Read the model definition and answer for the solid it produces. Units are mm, in the model's axes. Face numbers are marked on the shaded views. Round coordinates to 2 decimals unless told otherwise and drop trailing zeros. Write each loop counter-clockwise with the first axis right and the second up, starting at its lowest first coordinate (ties: lowest second). Pieces come first, ordered by that corner, then holes. Notation, with made-up numbers: (36.5, 17.5) -> (49.5, 17.5) arc R33 ccw to (49.5, 56.5) -> close; hole circle Ø1 at (-1, 77.25). An arc over 180 degrees is marked (long way). Return JSON: item names as keys, results as strings. Group by question number.
(1) Given pin 1 (1.1 mm diameter, centred on y = 10, z = -21, fed in from +X); pin 2 (8 mm diameter, centred on y = 10.5, z = -39, fed in from +X); pin 3 (8 mm diameter, centred on x = -22.5, y = 11.5, fed in from -Z), each flat-ended and moving along its own axis, determine where each tip first touches the part or whether it passes through.
(2) Straight lines are drawn through the part: line 1 (Z direction, x = -39.5, y = 1); line 2 (X direction, y = 2.1, z = 0); line 3 (X direction, y = 10.5, z = -7.5). For each, find the intervals that lie inside material, in ascending order.
(3) A cutting plane is placed at A-A on z = 0. Give the vertices of the cut face in (x, y), then the cut area to 3 significant figures.
(4) A cutting plane is placed at D-D on x = -20. Give the vertices of the cut face in (y, z).
(5) A cutting plane is placed at B-B on x = -40. Give the vertices of the cut face in (y, z), then the cut area to 3 significant figures.
(6) The mould has two halves that part along Y. Classify the marked faces 1 and 2: released by +Y, released by -Y, zero draft, split by the parting line, or undercut.
(7) A cutting plane is placed at C-C on z = 46.4. Give the vertices of the cut face in (x, y), then the cut area to 3 significant figures.
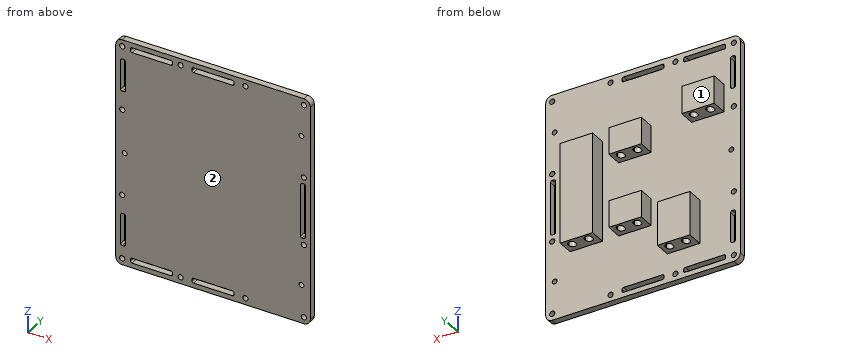
```python
from build123d import *

# Parameters (mm, degrees)
SKETCH1_W               = 120
SKETCH1_H               = 140
BOSS_EXTRUDE1_DEPTH     = 4
SKETCH2_R               = 1.6
CUT_EXTRUDE1_DEPTH      = 4
FILLET1_R               = 4
SKETCH5_W               = 20
SKETCH5_H               = 62
SKETCH5_H_2             = 27
BOSS_EXTRUDE2_DEPTH     = 10
SKETCH6_W               = 20
SKETCH6_H               = 10
SKETCH6_H_2             = 29
CUT_EXTRUDE3_DEPTH      = 10
CUT_EXTRUDE4_DEPTH      = 40
CUT_EXTRUDE4_DEPTH_BACK = 102
CUT_EXTRUDE5_DEPTH      = 20
CUT_EXTRUDE6_DEPTH      = 30
CUT_EXTRUDE7_DEPTH      = 5
SKETCH11_R              = 1.5
CUT_EXTRUDE8_DEPTH      = 5


with BuildPart() as part:
    # Sketch1 → Boss-Extrude1 (new body)
    with BuildSketch(Plane(origin=(0, 0, 0), x_dir=(1, 0, 0), z_dir=(0, 1, 0))):
        Rectangle(SKETCH1_W, SKETCH1_H)
    extrude(amount=BOSS_EXTRUDE1_DEPTH)

    # Sketch2 → Cut-Extrude1 (cut)
    with BuildSketch(Plane(origin=(0, 4, 0), x_dir=(1, 0, 0), z_dir=(0, 1, 0))):
        with Locations((-56, 66)):
            Circle(SKETCH2_R)
        with Locations((56, 66)):
            Circle(SKETCH2_R)
        with Locations((-56, -66)):
            Circle(SKETCH2_R)
        with Locations((56, -66)):
            Circle(SKETCH2_R)
        with Locations((-20, -66)):
            Circle(SKETCH2_R)
        with Locations((20, -66)):
            Circle(SKETCH2_R)
        with Locations((-20, 66)):
            Circle(SKETCH2_R)
        with Locations((20, 66)):
            Circle(SKETCH2_R)
        with Locations((-56, -26.5)):
            Circle(SKETCH2_R)
        with Locations((-56, 26.5)):
            Circle(SKETCH2_R)
        with Locations((56, -21)):
            Circle(SKETCH2_R)
        with Locations((56, 21)):
            Circle(SKETCH2_R)
    extrude(amount=-CUT_EXTRUDE1_DEPTH, mode=Mode.SUBTRACT)

    # Fillet1
    fillet1_edges = [part.edges().sort_by_distance(p)[0] for p in [
        (60, 2, 70),
        (-60, 2, 70),
        (-60, 2, -70),
        (60, 2, -70),
    ]]
    fillet(fillet1_edges, radius=FILLET1_R)

    # Sketch5 → Boss-Extrude2 (add)
    with BuildSketch(Plane(origin=(0, 4, 0), x_dir=(1, 0, 0), z_dir=(0, 1, 0))):
        with Locations((35, 0)):
            Rectangle(SKETCH5_W, SKETCH5_H)
        with Locations((-25, 38.5)):
            Rectangle(SKETCH5_W, SKETCH5_H_2)
        with Locations((5, 0)):
            Rectangle(SKETCH5_W, SKETCH5_H)
        with Locations((-40, -38.5)):
            Rectangle(SKETCH5_W, SKETCH5_H_2)
    extrude(amount=BOSS_EXTRUDE2_DEPTH)

    # Sketch6 → Cut-Extrude3 (cut)
    with BuildSketch(Plane(origin=(0, 14, 0), x_dir=(1, 0, 0), z_dir=(0, 1, 0))):
        with Locations((-40, -47)):
            Rectangle(SKETCH6_W, SKETCH6_H)
        with Locations((5, 0)):
            Rectangle(SKETCH6_W, SKETCH6_H_2)
    extrude(amount=-CUT_EXTRUDE3_DEPTH, mode=Mode.SUBTRACT)

    # Sketch7 → Cut-Extrude4 (cut, two sides)
    with BuildSketch(Plane.XY.offset(31)) as cut_extrude4_sk:
        with BuildLine():
            Line((-2.3, 9.4), (-2.3, 10.4))
            ThreePointArc((-2.3, 10.4), (-0.1, 12.6), (2.1, 10.4))
            Line((2.1, 10.4), (2.1, 9.4))
            ThreePointArc((2.1, 9.4), (-0.1, 7.2), (-2.3, 9.4))
        make_face()
        with BuildLine():
            Line((7.9, 9.4), (7.9, 10.4))
            ThreePointArc((7.9, 10.4), (10.1, 12.6), (12.3, 10.4))
            Line((12.3, 10.4), (12.3, 9.4))
            ThreePointArc((12.3, 9.4), (10.1, 7.2), (7.9, 9.4))
        make_face()
        with BuildLine():
            Line((27.7, 9.4), (27.7, 10.4))
            ThreePointArc((27.7, 10.4), (29.9, 12.6), (32.1, 10.4))
            Line((32.1, 10.4), (32.1, 9.4))
            ThreePointArc((32.1, 9.4), (29.9, 7.2), (27.7, 9.4))
        make_face()
        with BuildLine():
            Line((37.9, 9.4), (37.9, 10.4))
            ThreePointArc((37.9, 10.4), (40.1, 12.6), (42.3, 10.4))
            Line((42.3, 10.4), (42.3, 9.4))
            ThreePointArc((42.3, 9.4), (40.1, 7.2), (37.9, 9.4))
        make_face()
    extrude(amount=CUT_EXTRUDE4_DEPTH, mode=Mode.SUBTRACT)
    extrude(cut_extrude4_sk.sketch, amount=-CUT_EXTRUDE4_DEPTH_BACK, mode=Mode.SUBTRACT)

    # Sketch8 → Cut-Extrude5 (cut)
    with BuildSketch(Plane.XY.offset(42)):
        with BuildLine():
            Line((-47.3, 9.4), (-47.3, 10.4))
            ThreePointArc((-47.3, 10.4), (-45.1, 12.6), (-42.9, 10.4))
            Line((-42.9, 10.4), (-42.9, 9.4))
            ThreePointArc((-42.9, 9.4), (-45.1, 7.2), (-47.3, 9.4))
        make_face()
        with BuildLine():
            Line((-37.1, 9.4), (-37.1, 10.4))
            ThreePointArc((-37.1, 10.4), (-34.9, 12.6), (-32.7, 10.4))
            Line((-32.7, 10.4), (-32.7, 9.4))
            ThreePointArc((-32.7, 9.4), (-34.9, 7.2), (-37.1, 9.4))
        make_face()
    extrude(amount=-CUT_EXTRUDE5_DEPTH, mode=Mode.SUBTRACT)

    # Sketch9 → Cut-Extrude6 (cut)
    with BuildSketch(Plane(origin=(0, 0, -52), x_dir=(-1, 0, 0), z_dir=(0, 0, -1))):
        with BuildLine():
            Line((17.7, 9.4), (17.7, 10.4))
            ThreePointArc((17.7, 10.4), (19.9, 12.6), (22.1, 10.4))
            Line((22.1, 10.4), (22.1, 9.4))
            ThreePointArc((22.1, 9.4), (19.9, 7.2), (17.7, 9.4))
        make_face()
        with BuildLine():
            Line((27.9, 9.4), (27.9, 10.4))
            ThreePointArc((27.9, 10.4), (30.1, 12.6), (32.3, 10.4))
            Line((32.3, 10.4), (32.3, 9.4))
            ThreePointArc((32.3, 9.4), (30.1, 7.2), (27.9, 9.4))
        make_face()
    extrude(amount=-CUT_EXTRUDE6_DEPTH, mode=Mode.SUBTRACT)

    # Sketch10 → Cut-Extrude7 (cut, through all)
    with BuildSketch(Plane(origin=(0, 4, 0), x_dir=(1, 0, 0), z_dir=(0, 1, 0))):
        with BuildLine():
            Line((-56, 58), (-55, 58))
            ThreePointArc((-55, 58), (-54.292893219, 57.707106781), (-54, 57))
            Line((-54, 57), (-54, 39))
            ThreePointArc((-54, 39), (-54.292893219, 38.292893219), (-55, 38))
            Line((-55, 38), (-56, 38))
            ThreePointArc((-56, 38), (-56.707106781, 38.292893219), (-57, 39))
            Line((-57, 39), (-57, 57))
            ThreePointArc((-57, 57), (-56.707106781, 57.707106781), (-56, 58))
        make_face()
        with BuildLine():
            Line((-50, 67), (-26, 67))
            ThreePointArc((-26, 67), (-25.292893219, 66.707106781), (-25, 66))
            Line((-25, 66), (-25, 65))
            ThreePointArc((-25, 65), (-25.292893219, 64.292893219), (-26, 64))
            Line((-26, 64), (-50, 64))
            ThreePointArc((-50, 64), (-50.707106781, 64.292893219), (-51, 65))
            Line((-51, 65), (-51, 66))
            ThreePointArc((-51, 66), (-50.707106781, 66.707106781), (-50, 67))
        make_face()
        with BuildLine():
            Line((-12, 67), (12, 67))
            ThreePointArc((12, 67), (12.707106781, 66.707106781), (13, 66))
            Line((13, 66), (13, 65))
            ThreePointArc((13, 65), (12.707106781, 64.292893219), (12, 64))
            Line((12, 64), (-12, 64))
            ThreePointArc((-12, 64), (-12.707106781, 64.292893219), (-13, 65))
            Line((-13, 65), (-13, 66))
            ThreePointArc((-13, 66), (-12.707106781, 66.707106781), (-12, 67))
        make_face()
        with BuildLine():
            Line((55, 17), (56, 17))
            ThreePointArc((56, 17), (56.707106781, 16.707106781), (57, 16))
            Line((57, 16), (57, -16))
            ThreePointArc((57, -16), (56.707106781, -16.707106781), (56, -17))
            Line((56, -17), (55, -17))
            ThreePointArc((55, -17), (54.292893219, -16.707106781), (54, -16))
            Line((54, -16), (54, 16))
            ThreePointArc((54, 16), (54.292893219, 16.707106781), (55, 17))
        make_face()
    cut_extrude7 = extrude(amount=-CUT_EXTRUDE7_DEPTH, mode=Mode.SUBTRACT)

    # Mirror1: Cut-Extrude7 across plane
    add(cut_extrude7.mirror(Plane.XY), mode=Mode.SUBTRACT)

    # Sketch11 → Cut-Extrude8 (cut, through all)
    with BuildSketch(Plane(origin=(0, 4, 0), x_dir=(1, 0, 0), z_dir=(0, 1, 0))):
        with Locations((-54.5, 0)):
            Circle(SKETCH11_R)
        with Locations((54.5, -46.4)):
            Circle(SKETCH11_R)
        with Locations((54.5, 46.4)):
            Circle(SKETCH11_R)
    extrude(amount=-CUT_EXTRUDE8_DEPTH, mode=Mode.SUBTRACT)


solid = part.part
```
Checks:
{
 "1": {"pin 1": "stops at x = 45", "pin 2": "stops at x = -15", "pin 3": "stops at z = -52"},
 "2": {"line 1": "z = -70 to -67, -64 to 64, 67 to 70", "line 2": "x = -60 to -56, -53 to 54, 57 to 60", "line 3": "x = 25 to 27.7, 32.1 to 37.9, 42.3 to 45"},
 "3": {"outline": "(-60, 0) -> (-56, 0) -> (-56, 4) -> (-60, 4) -> close; (-53, 0) -> (54, 0) -> (54, 4) -> (45, 4) -> (45, 14) -> (25, 14) -> (25, 4) -> (-53, 4) -> close; (57, 0) -> (60, 0) -> (60, 4) -> (57, 4) -> close; hole (27.7, 9.4) arc R2.2 ccw to (32.1, 9.4) -> (32.1, 10.4) arc R2.2 ccw to (27.7, 10.4) -> close; hole (37.9, 9.4) arc R2.2 ccw to (42.3, 9.4) -> (42.3, 10.4) arc R2.2 ccw to (37.9, 10.4) -> close", "area": "617 mm^2"},
 "4": {"outline": "(0, -70) -> (4, -70) -> (4, -67.6) -> (0, -67.6) -> close; (0, -64.4) -> (4, -64.4) -> (4, -52) -> (7.2, -52) -> (7.2, -25) -> (4, -25) -> (4, 64.4) -> (0, 64.4) -> close; (0, 67.6) -> (4, 67.6) -> (4, 70) -> (0, 70) -> close; (12.6, -52) -> (14, -52) -> (14, -25) -> (12.6, -25) -> close"},
 "5": {"outline": "(0, -70) -> (4, -70) -> (4, -67) -> (0, -67) -> close; (0, -64) -> (4, -64) -> (4, 25) -> (14, 25) -> (14, 42) -> (4, 42) -> (4, 64) -> (0, 64) -> close; (0, 67) -> (4, 67) -> (4, 70) -> (0, 70) -> close", "area": "706 mm^2"},
 "6": {"face 1": "released by +Y", "face 2": "released by -Y"},
 "7": {"outline": "(-60, 0) -> (-57, 0) -> (-57, 4) -> (-60, 4) -> close; (-54, 0) -> (53, 0) -> (53, 4) -> (-54, 4) -> close; (56, 0) -> (60, 0) -> (60, 4) -> (56, 4) -> close", "area": "456 mm^2"}
}
